Build history of the part. All positions in model axes, mm. A direction names the side the tool comes from. Give positions to 0.01 mm unless a question says otherwise; leave off trailing zeros. Write each loop counter-clockwise with the first axis right and the second up, starting at its lowest first coordinate (ties: lowest second). Pieces come first, ordered by that corner, then holes.
from build123d import *

# Parameters (mm, degrees)
SKETCH1_W                                      = 105
SKETCH1_H                                      = 35
BOSS_EXTRUDE1_DEPTH                            = 5
M4_CLEARANCE_HOLE1_D                           = 4.5
SKETCH4_W                                      = 33.2
SKETCH4_H                                      = 35
BOSS_EXTRUDE2_DEPTH                            = 1.45
BOSS_EXTRUDE3_DEPTH                            = 17
CBORE_FOR_M2_5_SHCS1_AT_2_COUNT                = 2
CBORE_FOR_M2_5_SHCS1_AT_2_PITCH                = 12
CBORE_FOR_M2_5_SHCS1_AT_3_COUNT                = 2
CBORE_FOR_M2_5_SHCS1_AT_3_PITCH                = 24
CBORE_FOR_M2_5_SHCS1_AT_4_COUNT                = 2
CBORE_FOR_M2_5_SHCS1_AT_4_PITCH                = 26.83281573
BOSS_EXTRUDE5_DEPTH                            = 0.4
BOSS_EXTRUDE6_DEPTH                            = 0.4
CBORE_FOR_6_SOCKET_HEAD_CAP_SCREW1_D           = 3.997300108
CBORE_FOR_6_SOCKET_HEAD_CAP_SCREW1_CBORE_D     = 7.345020108
CBORE_FOR_6_SOCKET_HEAD_CAP_SCREW1_CBORE_DEPTH = 3.5052


with BuildPart() as part:
    # Sketch1 → Boss-Extrude1 (new body)
    with BuildSketch(Plane(origin=(0, 0, 0), x_dir=(1, 0, 0), z_dir=(0, 1, 0))):
        Rectangle(SKETCH1_W, SKETCH1_H)
    extrude(amount=BOSS_EXTRUDE1_DEPTH)

    # M4 Clearance Hole1 (through all)
    with Locations(Plane(origin=(0, 5, 0), x_dir=(1, 0, 0), z_dir=(0, 1, 0))):
        with Locations((-48.5, 7), (48.5, 7)):
            Hole(M4_CLEARANCE_HOLE1_D / 2)

    # Sketch4 → Boss-Extrude2 (add)
    with BuildSketch(Plane(origin=(0, 5, 0), x_dir=(1, 0, 0), z_dir=(0, 1, 0))):
        with Locations((-24.5, 0)):
            Rectangle(SKETCH4_W, SKETCH4_H)
    extrude(amount=BOSS_EXTRUDE2_DEPTH)

    # Sketch5 → Boss-Extrude3 (add, symmetric)
    with BuildSketch(Plane.ZY.offset(24.5)):
        Polygon((-17.5, 0), (-19.25, 0), (-19.25, 50.95), (-14.25, 50.95), (-14.25, 6.45), (-17.5, 6.45), align=None)
    boss_extrude3 = extrude(amount=BOSS_EXTRUDE3_DEPTH, both=True)

    # Sketch9 → CBORE for M2.5 SHCS1 (revolve, cut)
    with BuildSketch(Plane(origin=(-30.5, 45.7, -19.25), x_dir=(0, 1, 0), z_dir=(1, 0, 0))):
        Polygon((0, 0), (0, 34.490420021), (1.65, 33.499), (1.65, 4), (2.85, 4), (2.85, 0), align=None)
    cbore_for_m2_5_shcs1 = revolve(axis=Axis((-30.5, 45.7, -25.6), (0, 0, 1)), mode=Mode.SUBTRACT)

    # CBORE for M2.5 SHCS1 at 2: CBORE for M2.5 SHCS1 ×2
    with Locations(*[(i * CBORE_FOR_M2_5_SHCS1_AT_2_PITCH, 0, 0) for i in range(1, CBORE_FOR_M2_5_SHCS1_AT_2_COUNT)]):
        add(cbore_for_m2_5_shcs1, mode=Mode.SUBTRACT)

    # CBORE for M2.5 SHCS1 at 3: CBORE for M2.5 SHCS1 ×2
    with Locations(*[(0, -i * CBORE_FOR_M2_5_SHCS1_AT_3_PITCH, 0) for i in range(1, CBORE_FOR_M2_5_SHCS1_AT_3_COUNT)]):
        add(cbore_for_m2_5_shcs1, mode=Mode.SUBTRACT)

    # CBORE for M2.5 SHCS1 at 4: CBORE for M2.5 SHCS1 ×2
    with Locations(*[Vector(0.44721359549995815, -0.8944271909999159, 0) * (i * CBORE_FOR_M2_5_SHCS1_AT_4_PITCH) for i in range(1, CBORE_FOR_M2_5_SHCS1_AT_4_COUNT)]):
        add(cbore_for_m2_5_shcs1, mode=Mode.SUBTRACT)

    # Mirror1: Boss-Extrude3, CBORE for M2.5 SHCS1 across plane
    add(boss_extrude3.mirror(Plane(origin=(0, 0, 0), x_dir=(1, 0, 0), z_dir=(0, 0, -1))))
    add(cbore_for_m2_5_shcs1.mirror(Plane(origin=(0, 0, 0), x_dir=(1, 0, 0), z_dir=(0, 0, -1))), mode=Mode.SUBTRACT)

    # Mirror1 copy 1 sketch → Mirror1 copy 1 (revolve, cut)
    with BuildSketch(Plane(origin=(-18.5, 45.7, 19.25), x_dir=(0, 1, 0), z_dir=(1, 0, 0))):
        Polygon((0, 0), (0, -34.490420021), (1.65, -33.499), (1.65, -4), (2.85, -4), (2.85, 0), align=None)
    revolve(axis=Axis((-18.5, 45.7, 25.6), (0, 0, 1)), mode=Mode.SUBTRACT)

    # Mirror1 copy 2 sketch → Mirror1 copy 2 (revolve, cut)
    with BuildSketch(Plane(origin=(-30.5, 21.7, 19.25), x_dir=(0, 1, 0), z_dir=(1, 0, 0))):
        Polygon((0, 0), (0, -34.490420021), (1.65, -33.499), (1.65, -4), (2.85, -4), (2.85, 0), align=None)
    revolve(axis=Axis((-30.5, 21.7, 25.6), (0, 0, 1)), mode=Mode.SUBTRACT)

    # Mirror1 copy 3 sketch → Mirror1 copy 3 (revolve, cut)
    with BuildSketch(Plane(origin=(-18.5, 21.7, 19.25), x_dir=(0, 1, 0), z_dir=(1, 0, 0))):
        Polygon((0, 0), (0, -34.490420021), (1.65, -33.499), (1.65, -4), (2.85, -4), (2.85, 0), align=None)
    revolve(axis=Axis((-18.5, 21.7, 25.6), (0, 0, 1)), mode=Mode.SUBTRACT)

    # Sketch11 → Boss-Extrude5 (add)
    with BuildSketch(Plane(origin=(-7.9, 0, 0), x_dir=(0, 0, -1), z_dir=(1, 0, 0))):
        Polygon((17.5, 5), (17.5, 6.45), (14.25, 6.45), (-14.25, 6.45), (-17.5, 6.45), (-17.5, 5), align=None)
    extrude(amount=BOSS_EXTRUDE5_DEPTH)

    # Sketch12 → Boss-Extrude6 (add)
    with BuildSketch(Plane.ZY.offset(41.1)):
        Polygon((17.5, 5), (17.5, 6.45), (14.25, 6.45), (-14.25, 6.45), (-17.5, 6.45), (-17.5, 5), align=None)
    extrude(amount=BOSS_EXTRUDE6_DEPTH)

    # CBORE for #6 Socket Head Cap Screw1 (through all)
    with Locations(Plane(origin=(0, 0, 0), x_dir=(-1, 0, 0), z_dir=(0, -1, 0))):
        with Locations((-39.325, 9.779), (-11.514, 9.779), (-39.325, -9.639687995), (-11.514, -9.779)):
            CounterBoreHole(CBORE_FOR_6_SOCKET_HEAD_CAP_SCREW1_D / 2, CBORE_FOR_6_SOCKET_HEAD_CAP_SCREW1_CBORE_D / 2, CBORE_FOR_6_SOCKET_HEAD_CAP_SCREW1_CBORE_DEPTH)


solid = part.part
1. Drill centre lines: line 1 along X through (y, z) = (45.7, -16.55); line 2 along X through (y, z) = (21.7, -14.6); line 3 along Z through (x, y) = (-40, 48). Where is each one in solid material? Low to high.
2. Saw through at C-C on x = -30.5. Count the separate pieces of the cut face and the enclosed holes in it, plus the area to 3 significant figures.
3. Mould opens along Y. For faces 6 (the face through (-25, 50.95, -17)), 7 (the face through (-29, 44, -15.25)), 8 (the face through (-25, 25, 19.25)), 9 (the face through (-32.136, 45.485, 14.757)) say: pulls with the +Y half, pulls with the -Y half, needs draft (parallel to the pull), parting line crosses it, or undercut.
4. 3-axis set-ups, long thin cutter, end or side, ignore diameter. For faces 1 (the face through (22, 2, 17.5)), 2 (the face through (-24, 6.45, 0)), 3 (the face through (-29, 20, -15.25)), 4 (the face through (35.933, 1.728, -8.372)), 5 (the face through (-29, 44, 15.25)): which of +Z, -Z, +X, -X, +Y, -Y reach the whole face in a straight line?
5. Saw through at B-B on x = -48.5. Give the cut face in (y, z), plus the area to 4 significant figures.
6. Drop flat-ended pins along their axis: pin 1 (8.5 mm diameter, centred on x = 39.325, z = -9.779, fed in from +Y); pin 2 (5 mm diameter, centred on x = 39.33, z = 9.64, fed in from -Y); pin 3 (2.5 mm diameter, centred on x = 35, y = 1.5, fed in from +Z); pin 4 (1 mm diameter, centred on x = 27.5, y = 6.5, fed in from -Z). Give the stop position or say it passes through.
7. Saw through at A-A on y = 13.5. Give the cut face in (x, z), plus the area to 3 significant figures.
Outcome:
1. line 1: x = -41.5 to -33.35, -27.65 to -21.35, -15.65 to -7.5
1. line 2: x = -41.5 to -32.15, -28.85 to -20.15, -16.85 to -7.5
1. line 3: z = -19.25 to -14.25, 14.25 to 19.25
2. separate pieces: 5
2. enclosed holes: 0
2. area: 589 mm2
3. face 6: pulls with the +Y half
3. face 7: undercut
3. face 8: needs draft
3. face 9: undercut
4. face 1: +Z, +X, +Y, -Y
4. face 2: +X, -X, +Y
4. face 3: -Z
4. face 4: -Y
4. face 5: +Z
5. outline: (0, -17.5) - (5, -17.5) - (5, -9.25) - (0, -9.25) - close; (0, -4.75) - (5, -4.75) - (5, 17.5) - (0, 17.5) - close
5. area: 152.5 mm2
6. pin 1: stops at y = 5
6. pin 2: stops at y = 3.51
6. pin 3: stops at z = 17.5
6. pin 4: passes through
7. outline: (-41.5, -19.25) - (-7.5, -19.25) - (-7.5, -14.25) - (-41.5, -14.25) - close; (-41.5, 14.25) - (-7.5, 14.25) - (-7.5, 19.25) - (-41.5, 19.25) - close
7. area: 340 mm2
